```python
from build123d import *

# Parameters (mm, degrees)
SKETCH2_R           = 3.175
BOSS_EXTRUDE1_DEPTH = 0.254
SCALE1_SCALE        = 1.5
SCALE3_SCALE        = 1.5
SCALE5_SCALE        = 0.667


with BuildPart() as part:
    # Sketch2 → Boss-Extrude1 (new body)
    with BuildSketch(Plane.XY):
        with BuildLine():
            Line((6.35, 209.55), (6.35, 0))
            ThreePointArc((6.35, 0), (0, -6.35), (-6.35, 0))
            Line((-6.35, 0), (-6.35, 209.55))
            ThreePointArc((-6.35, 209.55), (0, 215.9), (6.35, 209.55))
        make_face()
        with Locations((0, 209.55)):
            Circle(SKETCH2_R, mode=Mode.SUBTRACT)
        Circle(SKETCH2_R, mode=Mode.SUBTRACT)
    extrude(amount=BOSS_EXTRUDE1_DEPTH)


with BuildPart() as part_1:
    # Scale1: scaled about (0, 104.775, 0.127)
    add(part.part.scale(SCALE1_SCALE).moved(Location((0, -52.3875, -0.0635))))


with BuildPart() as part_2:
    # Scale3: scaled about (0, 104.775, 0.127)
    add(part_1.part.scale(SCALE3_SCALE).moved(Location((0, -52.3875, -0.0635))))


with BuildPart() as part_3:
    # Scale5: scaled about (0, 104.775, 0.127)
    add(part_2.part.scale(SCALE5_SCALE).moved(Location((0, 34.890075, 0.042291))))


solid = part_3.part
```
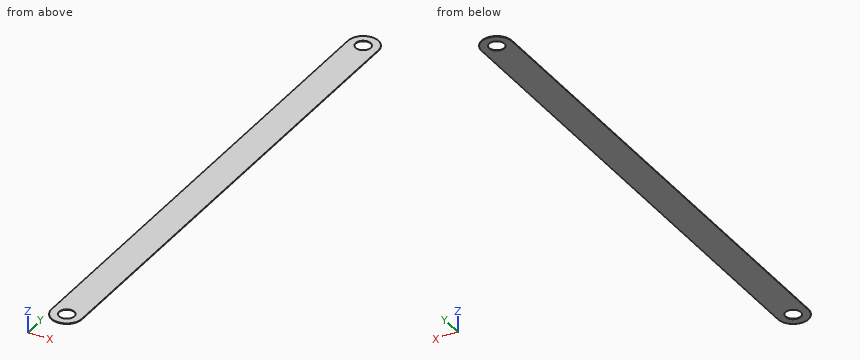
The model under review builds one solid part; all positions refer to its coordinate system, in mm. Give positions to 0.01 mm unless a question says otherwise; leave off trailing zeros. Write each loop counter-clockwise with the first axis right and the second up, starting at its lowest first coordinate (ties: lowest second). Pieces come first, ordered by that corner, then holes. Notation, with made-up numbers: (-15.75, 10.25) -> (0.25, 10.25) arc R20 ccw to (0.25, 31.25) -> close; hole circle Ø8 at (-3, -3). An arc over 180 degrees is marked (long way). Put each result on its own line as item: value.
(1) To check wall thickness, follow probe 1 along Y at (x, z) = (0, 0.05); probe 2 along Y at (x, z) = (-1.25, 0); probe 3 along Y at (x, z) = (-6.5, 0.05). State the ranges of each line that lie inside material, in increasing order. Write a range as from..to.
Results are:
probe 1: -62..-57.23, -47.7..257.25, 266.78..271.55
probe 2: -61.91..-57.06, -47.87..257.42, 266.61..271.46
probe 3: -59.44..268.99
(2) We need section A-A, the plane x = 0. Give the boundary of the cut face in (y, z).
Results are:
outline: (-62, -0.06) -> (-57.23, -0.06) -> (-57.23, 0.32) -> (-62, 0.32) -> close; (-47.7, -0.06) -> (257.25, -0.06) -> (257.25, 0.32) -> (-47.7, 0.32) -> close; (266.78, -0.06) -> (271.55, -0.06) -> (271.55, 0.32) -> (266.78, 0.32) -> close
(3) We need section B-B, the plane z = 0.05. Give the boundary of the cut face in (x, y), and give its area (3 significant figures).
Results are:
outline: (-9.53, -52.47) arc R9.53 ccw to (9.53, -52.47) -> (9.53, 262.02) arc R9.53 ccw to (-9.53, 262.02) -> close; hole circle Ø9.53 at (0, -52.47); hole circle Ø9.53 at (0, 262.02)
area: 6,140 mm²
(4) For pin 1 Ø8.5 at (x, y) = (0, -52.47) entering from +Z, flat-tipped, find the tip position at first contact; note if it passes through.
Results are:
pin 1: through
